```python
from build123d import *

# Parameters (mm, degrees)
SKETCH_1_R          = 3.5775
SKETCH_1_R_2        = 0.19875
EXTRUDE_2_DEPTH     = 0.159
EXTRUDE_START       = 0.3975
SKETCH_1_6_R        = 0.19875
EXTRUDE_3_DEPTH     = 0.3975
SCALE_2_SCALE       = 25
SKETCH_2_R          = 10
CUT_EXTRUDE_1_DEPTH = 23
SKETCH_3_W          = 10.6
SKETCH_3_H          = 6
CUT_EXTRUDE_2_DEPTH = 40


with BuildPart() as part:
    # Sketch 1 → Extrude 2 (new body)
    # profile 1 of 3: a face of its own
    with BuildSketch(Plane.XY):
        Circle(SKETCH_1_R)
        with Locations((-3.18, 0)):
            Circle(SKETCH_1_R_2, mode=Mode.SUBTRACT)
        with BuildLine():
            ThreePointArc((-1.985091803, -1.949799165), (2.7825, 0), (-1.985091803, 1.949799165))
            ThreePointArc((-1.985091803, 1.949799165), (-1.317199128, 0), (-1.985091803, -1.949799165))
        make_face(mode=Mode.SUBTRACT)
    # profile 2 of 3: a face of its own
    with BuildSketch(Plane.XY):
        with BuildLine():
            ThreePointArc((-1.985091803, -1.949799165), (-1.317199128, 0), (-1.985091803, 1.949799165))
            ThreePointArc((-1.985091803, 1.949799165), (2.7825, 0), (-1.985091803, -1.949799165))
        make_face()
        Circle(SKETCH_1_R_2, mode=Mode.SUBTRACT)
    # profile 3 of 3: a face of its own
    with BuildSketch(Plane.XY):
        with Locations((-3.18, 0)):
            Circle(SKETCH_1_R_2)
    extrude(amount=-EXTRUDE_2_DEPTH)

    # Sketch 1_6 → Extrude 3 (add)
    # profile 1 of 2: a face of its own
    with BuildSketch(Plane.XY.offset(EXTRUDE_START)):
        with BuildLine():
            ThreePointArc((-1.985091803, -1.949799165), (-1.317199128, 0), (-1.985091803, 1.949799165))
            ThreePointArc((-1.985091803, 1.949799165), (2.7825, 0), (-1.985091803, -1.949799165))
        make_face()
        Circle(SKETCH_1_6_R, mode=Mode.SUBTRACT)
    # profile 2 of 2: a face of its own
    with BuildSketch(Plane.XY.offset(EXTRUDE_START)):
        with Locations((-3.18, 0)):
            Circle(SKETCH_1_6_R)
    extrude(amount=-EXTRUDE_3_DEPTH)


with BuildPart() as part_1:
    # Scale 2: scaled about (0.208410277, 0, 0.076319073)
    add(part.part.scale(SCALE_2_SCALE).moved(Location((-5.001846648, 0, -1.831657752))))

    # Sketch 2 → Cut-Extrude 1 (cut)
    with BuildSketch(Plane.XY.offset(8.105842259)):
        with Locations((-5.001846653, 0)):
            Circle(SKETCH_2_R)
    extrude(amount=-CUT_EXTRUDE_1_DEPTH, mode=Mode.SUBTRACT)

    # Sketch 3 → Cut-Extrude 2 (cut)
    with BuildSketch(Plane.XY.offset(8.105842259)):
        with Locations((-15.001846653, 0)):
            Rectangle(SKETCH_3_W, SKETCH_3_H)
    extrude(amount=-CUT_EXTRUDE_2_DEPTH, mode=Mode.SUBTRACT)


solid = part_1.part
```
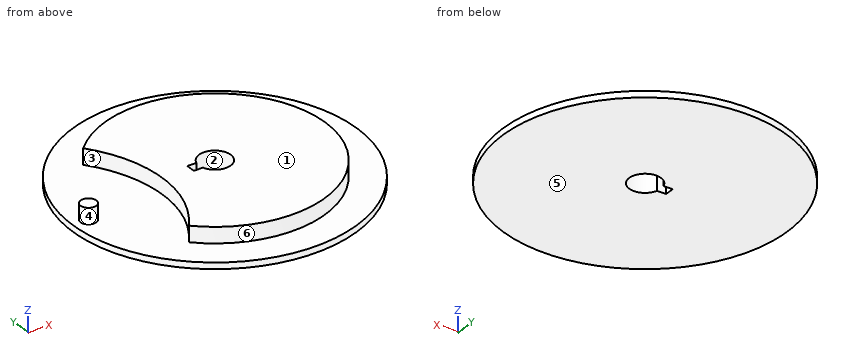
Model file for the job. Use its own axes, mm. Face numbers are marked on the shaded views. A direction names the side the tool comes from. Give positions to 0.01 mm unless a question says otherwise; leave off trailing zeros. Loops run counter-clockwise (first coordinate to the right, second up) from the corner with the lowest first, then second, coordinate; pieces in that order, holes last. Notation, with made-up numbers: (49, 4.25) -> (85, 4.25) arc R20 ccw to (85, 32.25) -> close; hole circle Ø6 at (16, 39). An arc over 180 degrees is marked (long way). Use CSV: the item, a comma, the result in double quotes. Start each with the question number.
1) Slice it at B-B on y = 0. Give the cut face in (x, z), plus the area to 3 significant figures.
2) Wall check: line 1 (Y direction, x = -4, z = 6.75); line 2 (Z direction, x = 58, y = -40); line 3 (Y direction, x = 3.5, z = 2.5). Give the ranges that are in metal, low to high.
3) Slice it at D-D on y = 55.5. Give the cut face in (x, z).
4) Mould opens along Y. For the marked faces 1, 2, 3 and 4 say: released by +Y, released by -Y, zero draft, split by the parting line, or undercut.
5) Tool access for the marked faces 5 and 6: list every direction of +Z, -Z, +X, -X, +Y, -Y with a clear straight run to the whole face (end or side of a thin tool).
6) Slice it at A-A on z = 5. Give the cut face in (x, y) (1 decimal), plus the area to 3 significant figures.
7) Flat gauge pins, fed straight in: pin 1 Ø1.7 at (x, z) = (-16, 0.5) entering from +Y; pin 2 Ø2 at (y, z) = (30, -0.5) entering from -X; pin 3 Ø6 at (x, z) = (-38, 3.5) entering from -Y. Where does each tip first touch, or does it go through?
8) Slice it at C-C on x = -30.5. Give the cut face in (y, z), plus the area to 3 significant figures.
Computed values:
1,outline,"(-94.44, -5.81) -> (-20.3, -5.81) -> (-20.3, 8.11) -> (-37.93, 8.11) -> (-37.93, -1.83) -> (-79.53, -1.83) -> (-79.53, 8.11) -> (-89.47, 8.11) -> (-89.47, -1.83) -> (-94.44, -1.83) -> close; (5, -5.81) -> (84.44, -5.81) -> (84.44, -1.83) -> (64.56, -1.83) -> (64.56, 8.11) -> (5, 8.11) -> close"
1,area,"1,480 mm^2"
2,line 1,"y = -69.56 to -9.95, 9.95 to 69.56"
2,line 2,"z = -5.81 to -1.83"
2,line 3,"y = -69.04 to -5.26, 5.26 to 69.04"
3,outline,"(-75.14, -5.81) -> (65.13, -5.81) -> (65.13, -1.83) -> (36.93, -1.83) -> (36.93, 8.11) -> (-46.94, 8.11) -> (-46.94, -1.83) -> (-75.14, -1.83) -> close"
4,face 1,"zero draft"
4,face 2,"undercut"
4,face 3,"undercut"
4,face 4,"split by the parting line"
5,face 5,"-Z, +X, -X, +Y, -Y"
5,face 6,"+Z"
6,outline,"circle Ø9.9 at (-84.5, 0); (-54.6, -48.7) arc R69.6 ccw (long way) to (-54.6, 48.7) arc R79.5 cw to start; hole (-20.3, -3) -> (-14.5, -3) arc R10 ccw (long way) to (-14.5, 3) -> (-20.3, 3) -> close"
6,area,"12,500 mm^2"
7,pin 1,"stops at y = 68.82"
7,pin 2,"stops at x = -44.22"
7,pin 3,"stops at y = -62.76"
8,outline,"(-85.73, -5.81) -> (85.73, -5.81) -> (85.73, -1.83) -> (64.72, -1.83) -> (64.72, 8.11) -> (-64.72, 8.11) -> (-64.72, -1.83) -> (-85.73, -1.83) -> close"
8,area,"1,970 mm^2"
